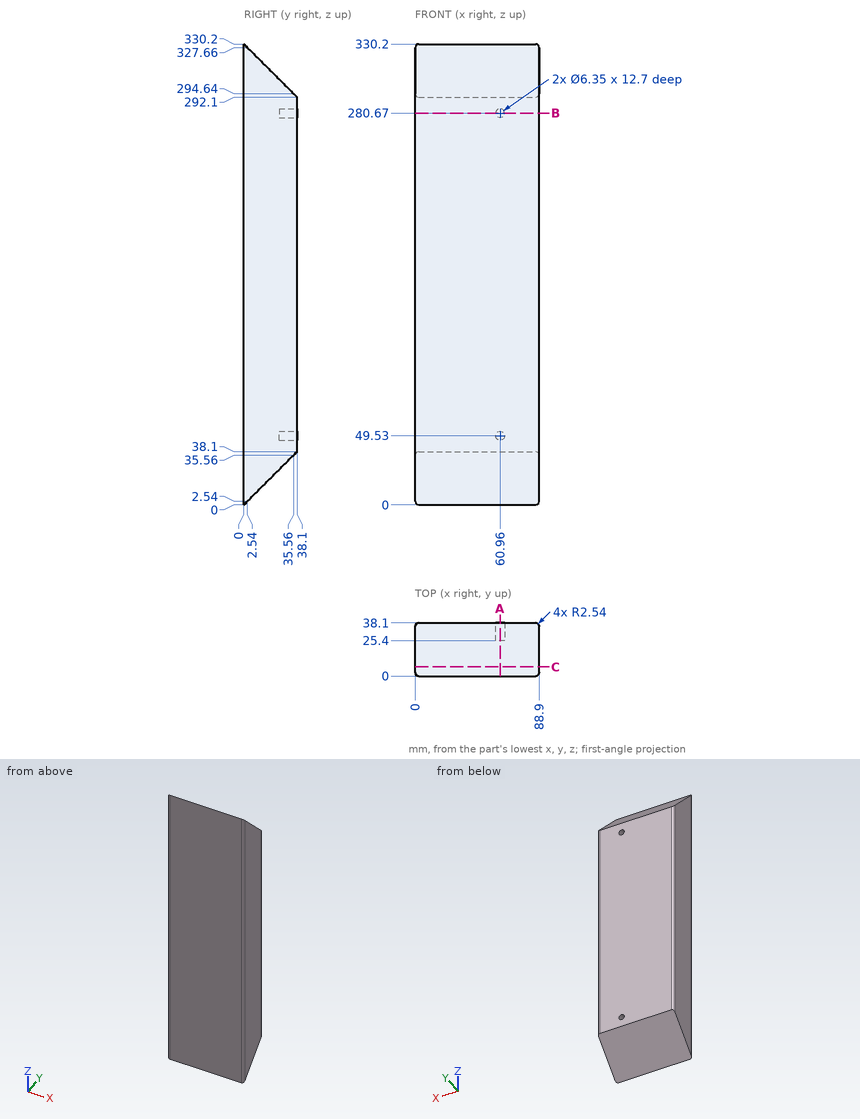
Input: dimensioned drawing with shaded views. Units: mm. Origin: part minimum x, y, z. Round coordinates to 2 decimals unless told otherwise and drop trailing zeros. Order: outer loops, then holes, each group sorted by start corner. A loop starts at its lowest first (then second) coordinate and runs counter-clockwise, first axis right, second up.
Q1. Section C-C, the plane y = 6.5. Output: boundary loops of the cut face in (x, z).
Result sheet:
outline: (0, 6.5) - (88.9, 6.5) - (88.9, 323.7) - (0, 323.7) - close
Q2. Section A-A, the plane x = 60.96. Output: boundary loops of the cut face in (y, z) (3 decimals).
Result sheet:
outline: (0, 0) - (38.1, 38.1) - (38.1, 46.355) - (25.4, 46.355) - (25.4, 52.705) - (38.1, 52.705) - (38.1, 277.495) - (25.4, 277.495) - (25.4, 283.845) - (38.1, 283.845) - (38.1, 292.1) - (0, 330.2) - close
Q3. Material intervals for probe 1 along X at (y, z) = (33, 49.53) (3 decimals); probe 2 along Z at (x, y) = (60, 35); probe 3 along Z at (x, y) = (60.96, 31.75) (3 decimals), sorted ascending.
Result sheet:
probe 1: x = 0 to 57.785, 64.135 to 88.9
probe 2: z = 35 to 46.5, 52.56 to 277.64, 283.7 to 295.2
probe 3: z = 31.75 to 46.355, 52.705 to 277.495, 283.845 to 298.45
Q4. Section B-B, the plane z = 280.67. Output: boundary loops of the cut face in (x, y) (3 decimals), and give its area (3 significant figures).
Result sheet:
outline: (0, 2.54) arc R2.54 ccw to (2.54, 0) - (86.36, 0) arc R2.54 ccw to (88.9, 2.54) - (88.9, 35.56) arc R2.54 ccw to (86.36, 38.1) - (64.135, 38.1) - (64.135, 25.4) - (57.785, 25.4) - (57.785, 38.1) - (2.54, 38.1) arc R2.54 ccw to (0, 35.56) - close
area: 3,300 mm2
Q5. Pin query (flat end, axial travel): pin 1 (5 mm diameter, centred on x = 9.5, y = 15, fed in from -Z); pin 2 (1.5 mm diameter, centred on x = 10, y = 20, fed in from +Z); pin 3 (5 mm diameter, centred on x = 18.5, z = 35, fed in from +Y). Return the tip coordinate at first contact, or that it passes through.
Result sheet:
pin 1: stops at z = 12.5
pin 2: stops at z = 310.95
pin 3: stops at y = 37.5
